from build123d import *

# Parameters (mm, degrees)
EXTRUDE_THIN1_DEPTH = 38
CUT_EXTRUDE1_DEPTH  = 4
CUT_EXTRUDE2_DEPTH  = 4


with BuildPart() as part:
    # Sketch1 → Extrude-Thin1 (new body)
    with BuildSketch(Plane.XY):
        Polygon((0, 20), (0, 0), (20, 0), (20, 3), (3, 3), (3, 20), align=None)
    extrude(amount=EXTRUDE_THIN1_DEPTH)

    # Sketch2 → Cut-Extrude1 (cut, through all)
    with BuildSketch(Plane(origin=(3, 0, 0), x_dir=(0, 0, -1), z_dir=(1, 0, 0))):
        with BuildLine():
            Line((-29, 7.25), (-32.5, 7.25))
            ThreePointArc((-32.5, 7.25), (-35.25, 10), (-32.5, 12.75))
            Line((-32.5, 12.75), (-29, 12.75))
            ThreePointArc((-29, 12.75), (-26.25, 10), (-29, 7.25))
        make_face()
        with BuildLine():
            Line((-9, 7.25), (-5.5, 7.25))
            ThreePointArc((-5.5, 7.25), (-2.75, 10), (-5.5, 12.75))
            Line((-5.5, 12.75), (-9, 12.75))
            ThreePointArc((-9, 12.75), (-11.75, 10), (-9, 7.25))
        make_face()
    extrude(amount=-CUT_EXTRUDE1_DEPTH, mode=Mode.SUBTRACT)

    # Sketch3 → Cut-Extrude2 (cut, through all)
    with BuildSketch(Plane(origin=(0, 3, 0), x_dir=(1, 0, 0), z_dir=(0, 1, 0))):
        with BuildLine():
            Line((12.25, -32.5), (12.25, -29))
            ThreePointArc((12.25, -29), (15, -26.25), (17.75, -29))
            Line((17.75, -29), (17.75, -32.5))
            ThreePointArc((17.75, -32.5), (15, -35.25), (12.25, -32.5))
        make_face()
        with BuildLine():
            Line((12.25, -5.5), (12.25, -9))
            ThreePointArc((12.25, -9), (15, -11.75), (17.75, -9))
            Line((17.75, -9), (17.75, -5.5))
            ThreePointArc((17.75, -5.5), (15, -2.75), (12.25, -5.5))
        make_face()
    extrude(amount=-CUT_EXTRUDE2_DEPTH, mode=Mode.SUBTRACT)


solid = part.part
The listing builds one solid part. Answer for the finished solid, in the listing's coordinates (mm). A direction names the side the tool comes from. Round coordinates to 2 decimals unless told otherwise and drop trailing zeros. Write each loop counter-clockwise with the first axis right and the second up, starting at its lowest first coordinate (ties: lowest second). Pieces come first, ordered by that corner, then holes. Notation, with made-up numbers: M 13.5,86.25 L 44.5,86.25 A25 cw 44.5,105.25 Z; hole C 31.25,53 d4. An arc over 180 degrees is marked long. Write each question's results on one line, items separated by ' | '. Start each with the question number.
Item 1: A cutting plane is placed at A-A on y = 10. Write down the section's boundary in (x, z), and give its area (3 significant figures).
Item 2: For a pull along Z with two mould halves and no side action, classify faces 4 (the face through (17.75, 2, 31)), 5 (the face through (3, 11, 19)), 6 (the face through (2.5, 6.3, 0)) as pulls with the +Z half, pulls with the -Z half, needs draft (parallel to the pull), parting line crosses it, or undercut.
Item 3: A cutting plane is placed at B-B on z = 31. Write down the section's boundary in (x, y).
Item 4: For faces 1 (the face through (2, 12.75, 7)), 2 (the face through (20, 1, 19)), 3 (the face through (14.94, 1.52, 11.75)), determine the directions among +Z, -Z, +X, -X, +Y, -Y from which every point of the face is accessible in a straight line to the end or side of a thin tool.
Item 5: Straight lines are drawn through the part: L1, parallel to X at y = 1, z = 9; L2, parallel to X at y = 18.25, z = 30.5. For each, find the intervals that lie inside material, in ascending order. Write a range as [from, to].
Item 6: Flat-ended cylindrical pins translate along their axes: pin 1 Ø1.5 at (x, z) = (14, 15.5) entering from -Y; pin 2 Ø1 at (y, z) = (6, 26) entering from +X. Find the tip coordinate at first contact, or state that the pin passes through.
Item 7: A cutting plane is placed at D-D on x = 11.75. Write down the section's boundary in (y, z), and give its area (3 significant figures).
Check sheet entries:
1) outline: M 0,0 L 3,0 L 3,2.75 L 0,2.75 Z; M 0,11.75 L 3,11.75 L 3,26.25 L 0,26.25 Z; M 0,35.25 L 3,35.25 L 3,38 L 0,38 Z | area: 60.0 mm²
2) face 4: undercut | face 5: needs draft | face 6: pulls with the -Z half
3) outline: M 0,0 L 12.25,0 L 12.25,3 L 3,3 L 3,7.25 L 0,7.25 Z; M 0,12.75 L 3,12.75 L 3,20 L 0,20 Z; M 17.75,0 L 20,0 L 20,3 L 17.75,3 Z
4) face 1: +X, -X | face 2: +Z, -Z, +X, +Y, -Y | face 3: +Y, -Y
5) L1: [0, 12.25], [17.75, 20] | L2: [0, 3]
6) pin 1: y = 0 | pin 2: x = 3
7) outline: M 0,0 L 3,0 L 3,38 L 0,38 Z | area: 114 mm²
